```python
from build123d import *

# Parameters (mm, degrees)
F1_DEPTH      = 20
F1_DEPTH_BACK = 5
F3_DEPTH      = 5
F7_DEPTH      = 80


with BuildPart() as f1:
    # F0 (on Front) → F1 (new body, two sides)
    with BuildSketch(Plane.XZ) as f1_sk:
        with BuildLine():
            Line((0, 17), (0, 25))
            ThreePointArc((0, 25), (-25, 0), (0, -25))
            Line((0, -25), (0, -17))
            ThreePointArc((0, -17), (-17, 0), (0, 17))
        make_face()
    extrude(amount=F1_DEPTH)
    extrude(f1_sk.sketch, amount=-F1_DEPTH_BACK)

    # F2 (on Front) → F3 (join)
    with BuildSketch(Plane.XZ):
        with BuildLine():
            Line((-65, 77), (-65, 32.1130814467))
            ThreePointArc((-65, 32.1130814467), (-61.5810376857, -38.2625900529), (0, -72.5))
            Line((0, -72.5), (0, -25))
            ThreePointArc((0, -25), (-25, 0), (0, 25))
            Line((0, 25), (0, 77))
            Line((0, 77), (-65, 77))
        make_face()
    extrude(amount=-F3_DEPTH)


with BuildPart() as f5_1:
    # F5: instance of F1
    add(f1.part.mirror(Plane.XZ.offset(40)))


with BuildPart() as f1_1:
    add(f1.part)

    add(f5_1.part)  # F7 merges F5_1
    # F6 (on face) → F7 (join, through all)
    with BuildSketch(Plane.XZ):
        with BuildLine():
            Line((-65, 77), (-65, 32.1130814467))
            ThreePointArc((-65, 32.1130814467), (-61.5810376857, -38.2625900529), (0, -72.5))
            Line((0, -72.5), (0, -68.0532879441))
            ThreePointArc((0, -68.0532879441), (-58.3808649236, -34.9703390142), (-60, 32.1130814467))
            Line((-60, 32.1130814467), (-60, 77))
            Line((-60, 77), (-65, 77))
        make_face()
    extrude(amount=F7_DEPTH)


solid = f1_1.part
```
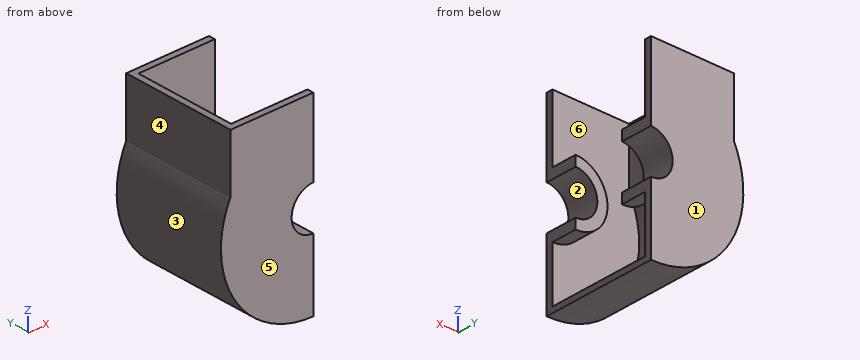
CAD build for the part. Positions are in the model's coordinates, mm. Face numbers are marked on the shaded views. A direction names the side the tool comes from. Give positions to 0.01 mm unless a question says otherwise; leave off trailing zeros. Order: outer loops, then holes, each group sorted by start corner. A loop starts at its lowest first (then second) coordinate and runs counter-clockwise, first axis right, second up.
(1) Saw through at B-B, the plane z = 50. Give the cut face in (x, y).
(2) Saw through at A-A, the plane y = -64. Give the cut face in (x, z).
(3) Saw through at C-C, the plane x = -23. Give the cut face in (y, z) (3 decimals).
(4) Mould opens along Z. For the marked faces 1, 2 and 3 say: released by +Z, released by -Z, zero draft, split by the parting line, or undercut.
(5) Saw through at D-D, the plane y = -41. Give the cut face in (x, z), then the cut area to 3 significant figures.
(6) Flat gauge pins, fed straight in: pin 1 (2 mm diameter, centred on y = -13, z = 17, fed in from -X); pin 2 (22.5 mm diameter, centred on y = -37.5, z = 62, fed in from -X); pin 3 (1.5 mm diameter, centred on x = -29.5, y = -5.5, fed in from +Z). Where does each tip first touch, or does it go through?
(7) Tool access for the marked faces 4, 5 and 6: list every direction of +Z, -Z, +X, -X, +Y, -Y with a clear straight run to the whole face (end or side of a thin tool).
(8) Drill centre lines: L1, parallel to Y at x = -10.5, z = -44.5; L2, parallel to Z at x = -4.5, y = -62.5; L3, parallel to Z at x = -9, y = -4. Where is each one in solid material? Low to high.
Results found:
1. outline: (-65, -85) - (0, -85) - (0, -80) - (-60, -80) - (-60, 0) - (0, 0) - (0, 5) - (-65, 5) - close
2. outline: (-65, 32.11) arc R72.5 ccw to (0, -72.5) - (0, -68.05) arc R68.05 cw to (-60, 32.11) - (-60, 77) - (-65, 77) - close; (0, -25) - (0, -17) arc R17 cw to (0, 17) - (0, 25) arc R25 ccw to start
3. outline: (-85, -68.755) - (5, -68.755) - (5, 77) - (0, 77) - (0, 9.798) - (-20, 9.798) - (-20, -9.798) - (0, -9.798) - (0, -64.049) - (-80, -64.049) - (-80, -9.798) - (-60, -9.798) - (-60, 9.798) - (-80, 9.798) - (-80, 77) - (-85, 77) - close
4. face 1: zero draft
4. face 2: undercut
4. face 3: split by the parting line
5. outline: (-65, 32.11) arc R72.5 ccw to (0, -72.5) - (0, -68.05) arc R68.05 cw to (-60, 32.11) - (-60, 77) - (-65, 77) - close
5. area: 864 mm2
6. pin 1: stops at x = -70.71
6. pin 2: stops at x = -65
6. pin 3: stops at z = -60.96
7. face 4: +Z, -X, +Y, -Y
7. face 5: +Z, -Z, +X, -X, -Y
7. face 6: none
8. L1: y = -85 to -80, 0 to 5
8. L2: z = -72.36 to -67.9, -24.59 to -16.39, 16.39 to 24.59
8. L3: z = -71.94 to -67.46, -23.32 to -14.42, 14.42 to 23.32
